Geometry check sheet. Reference: the model listing, model coordinates, mm. Face numbers are marked on the shaded views. Round coordinates to 2 decimals unless told otherwise and drop trailing zeros. Order: outer loops, then holes, each group sorted by start corner. A loop starts at its lowest first (then second) coordinate and runs counter-clockwise, first axis right, second up. Notation, with made-up numbers: (85, -37) - (96, -37) arc R16 cw to (96, -17) - close; hole circle Ø2 at (-7, -28). An arc over 180 degrees is marked (long way). Write each question's results on one line, items separated by ' | '.
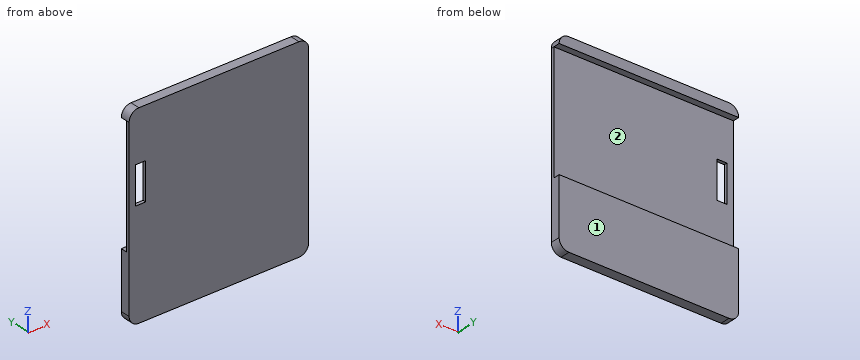
```python
from build123d import *

# Parameters (mm, degrees)
BOSS_EXTRUDE1_DEPTH   = 3
BOSS_EXTRUDE1_2_DEPTH = 3
SKETCH1_5_W           = 55.2
SKETCH1_5_H           = 36.5
SKETCH1_5_W_2         = 3.1
SKETCH1_5_H_2         = 11.5
BOSS_EXTRUDE2_DEPTH   = 1


with BuildPart() as part:
    # Sketch1 → Boss-Extrude1 (new body)
    with BuildSketch(Plane(origin=(0, 0, 0), x_dir=(1, 0, 0), z_dir=(0, 1, 0))):
        with BuildLine():
            ThreePointArc((-24.6, -30), (-26.721320344, -29.121320344), (-27.6, -27))
            Line((-27.6, -27), (27.6, -27))
            ThreePointArc((27.6, -27), (26.721320344, -29.121320344), (24.6, -30))
            Line((24.6, -30), (-24.6, -30))
        make_face()
    extrude(amount=BOSS_EXTRUDE1_DEPTH)



with BuildPart() as body_2:
    # Sketch1 → Boss-Extrude1 2 (new body)
    with BuildSketch(Plane(origin=(0, 0, 0), x_dir=(1, 0, 0), z_dir=(0, 1, 0))):
        with BuildLine():
            Line((-27.6, 27), (-27.6, 9.5))
            Line((-27.6, 9.5), (27.6, 9.5))
            Line((27.6, 9.5), (27.6, 27))
            ThreePointArc((27.6, 27), (26.721320344, 29.121320344), (24.6, 30))
            Line((24.6, 30), (-24.6, 30))
            ThreePointArc((-24.6, 30), (-26.721320344, 29.121320344), (-27.6, 27))
        make_face()
    extrude(amount=BOSS_EXTRUDE1_2_DEPTH)


with BuildPart() as part_1:
    add(part.part)

    add(body_2.part)  # Boss-Extrude2 merges body 2
    # Sketch1_5 → Boss-Extrude2 (add)
    with BuildSketch(Plane(origin=(0, 0, 0), x_dir=(1, 0, 0), z_dir=(0, 1, 0))):
        with Locations((0, -8.75)):
            Rectangle(SKETCH1_5_W, SKETCH1_5_H)
        with Locations((-24.05, -8.75)):
            Rectangle(SKETCH1_5_W_2, SKETCH1_5_H_2, mode=Mode.SUBTRACT)
    extrude(amount=BOSS_EXTRUDE2_DEPTH)


solid = part_1.part
```
(1) Depth check by flat-ended pin: pin 1 Ø4 at (x, z) = (5, 13) entering from +Y; pin 2 Ø1 at (y, z) = (2, 8.5) entering from +X. Enter the tip coordinate at first touch or a pass-through.
Answers follow:
pin 1: y = 1 | pin 2: through
(2) Section check B-B (z = 10). Record the cut outline in (x, y).
Answers follow:
outline: (-27.6, 0) - (-25.6, 0) - (-25.6, 1) - (-27.6, 1) - close; (-22.5, 0) - (27.6, 0) - (27.6, 1) - (-22.5, 1) - close
(3) Section check D-D (z = 17). Record the cut outline in (x, y).
Answers follow:
outline: (-27.6, 0) - (27.6, 0) - (27.6, 1) - (-27.6, 1) - close
(4) Material ranges on line 1 (Z direction, x = -3.5, y = 2.05); line 2 (Y direction, x = -4, z = 9.5); line 3 (X direction, y = 0.7, z = 27.5), recorded low to high.
Answers follow:
line 1: -30 to -9.5, 27 to 30 | line 2: 0 to 1 | line 3: -27.56 to 27.56
(5) Section check A-A (y = 2.1). Record the cut outline in (x, z), then the cut area to 3 significant figures.
Answers follow:
outline: (-27.6, -27) arc R3 ccw to (-24.6, -30) - (24.6, -30) arc R3 ccw to (27.6, -27) - (27.6, -9.5) - (-27.6, -9.5) - close; (-27.6, 27) - (27.6, 27) arc R3 ccw to (24.6, 30) - (-24.6, 30) arc R3 ccw to start | area: 1,290 mm²
(6) Section check C-C (x = -10). Record the cut outline in (y, z).
Answers follow:
outline: (0, -30) - (3, -30) - (3, -9.5) - (1, -9.5) - (1, 27) - (3, 27) - (3, 30) - (0, 30) - close
(7) Draft check along Z on the marked faces 1 and 2. Enter one of: released by +Z, released by -Z, zero draft, split by the parting line, or undercut.
Answers follow:
face 1: zero draft | face 2: undercut
